Verification items for the finished model (mm, model axes). Round coordinates to 2 decimals unless told otherwise and drop trailing zeros. Order: outer loops, then holes, each group sorted by start corner. A loop starts at its lowest first (then second) coordinate and runs counter-clockwise, first axis right, second up. Notation, with made-up numbers: (45, 81) -> (84, 81) arc R33 cw to (84, 114) -> close; hole circle Ø10 at (-14.75, 15.5). An arc over 180 degrees is marked (long way). Return JSON: item names as keys, results as strings. Group by question number.
1) Scan lines: L1, parallel to Z at x = -3, y = 86.5; L2, parallel to X at y = 77, z = -0.7; L3, parallel to Z at x = 1.5, y = 138.5. Record each from-to range of solid material in increasing order.
2) Depth check by flat-ended pin: pin 1 (2.5 mm diameter, centred on x = 0, y = 155, fed in from -Z); pin 2 (1 mm diameter, centred on y = 116.5, z = -2, fed in from -X); pin 3 (0.5 mm diameter, centred on y = 141, z = -1, fed in from -X). Enter the tip coordinate at first touch or a pass-through.
3) Section check A-A on y = 115.5. Enter the section's corners in (x, z), plus the area to 3 significant figures.
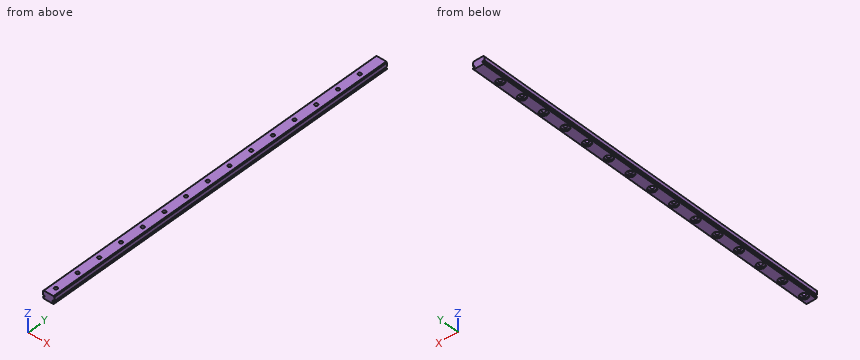
```python
from build123d import *

# Parameters (mm, degrees)
EXTRUDE_1_DEPTH     = 230
SKETCH_2_R          = 1
CUT_EXTRUDE_1_DEPTH = 10
CHAMFER_1_SIZE      = 0.5
SKETCH_3_R          = 2.383304988
CUT_EXTRUDE_2_DEPTH = 1


with BuildPart() as part:
    # 草图1 → 凸台-拉伸1 (new body)
    with BuildSketch(Plane(origin=(0, 0, 0), x_dir=(1, 0, 0), z_dir=(0, 1, 0))):
        Polygon((-3.5, 0.4), (-3.5, -2.4), (3.5, -2.4), (3.5, 0.4), (2.5, 0.4), (2.5, 1.4), (3.5, 1.4), (3.5, 2.4), (-3.5, 2.4), (-3.5, 1.4), (-2.5, 1.4), (-2.5, 0.4), align=None)
    extrude(amount=EXTRUDE_1_DEPTH)

    # 草图2 → 切除-拉伸1 (cut)
    with BuildSketch(Plane(origin=(0, 0, -2.4), x_dir=(-1, 0, 0), z_dir=(0, 0, -1))):
        with Locations((0, 5)):
            Circle(SKETCH_2_R)
        with Locations((0, 20)):
            Circle(SKETCH_2_R)
        with Locations((0, 35)):
            Circle(SKETCH_2_R)
        with Locations((0, 50)):
            Circle(SKETCH_2_R)
        with Locations((0, 65)):
            Circle(SKETCH_2_R)
        with Locations((0, 80)):
            Circle(SKETCH_2_R)
        with Locations((0, 95)):
            Circle(SKETCH_2_R)
        with Locations((0, 110)):
            Circle(SKETCH_2_R)
        with Locations((0, 125)):
            Circle(SKETCH_2_R)
        with Locations((0, 140)):
            Circle(SKETCH_2_R)
        with Locations((0, 155)):
            Circle(SKETCH_2_R)
        with Locations((0, 170)):
            Circle(SKETCH_2_R)
        with Locations((0, 185)):
            Circle(SKETCH_2_R)
        with Locations((0, 200)):
            Circle(SKETCH_2_R)
        with Locations((0, 215)):
            Circle(SKETCH_2_R)
    extrude(amount=-CUT_EXTRUDE_1_DEPTH, mode=Mode.SUBTRACT)

    # 倒角1
    chamfer_1_edges = [part.edges().sort_by_distance(p)[0] for p in [
        (-3.5, 115, -2.4),
        (3.5, 115, -2.4),
        (3.5, 115, 2.4),
        (-3.5, 115, 2.4),
    ]]
    chamfer(chamfer_1_edges, length=CHAMFER_1_SIZE)

    # 草图3 → 切除-拉伸2 (cut)
    with BuildSketch(Plane(origin=(0, 0, -2.4), x_dir=(-1, 0, 0), z_dir=(0, 0, -1))):
        with Locations((0, 5)):
            Circle(SKETCH_3_R)
        with Locations((0, 20)):
            Circle(SKETCH_3_R)
        with Locations((0, 35)):
            Circle(SKETCH_3_R)
        with Locations((0, 50)):
            Circle(SKETCH_3_R)
        with Locations((0, 65)):
            Circle(SKETCH_3_R)
        with Locations((0, 80)):
            Circle(SKETCH_3_R)
        with Locations((0, 95)):
            Circle(SKETCH_3_R)
        with Locations((0, 110)):
            Circle(SKETCH_3_R)
        with Locations((0, 125)):
            Circle(SKETCH_3_R)
        with Locations((0, 140)):
            Circle(SKETCH_3_R)
        with Locations((0, 155)):
            Circle(SKETCH_3_R)
        with Locations((0, 170)):
            Circle(SKETCH_3_R)
        with Locations((0, 185)):
            Circle(SKETCH_3_R)
        with Locations((0, 200)):
            Circle(SKETCH_3_R)
        with Locations((0, 215)):
            Circle(SKETCH_3_R)
    extrude(amount=-CUT_EXTRUDE_2_DEPTH, mode=Mode.SUBTRACT)


solid = part.part
```
Check result:
{
 "1": {"L1": "-2.4 to -1.4, -0.4 to 2.4", "L2": "-2.5 to 2.5", "L3": "-1.4 to 2.4"},
 "2": {"pin 1": "z = -1.4", "pin 2": "x = -3.5", "pin 3": "x = -2.5"},
 "3": {"outline": "(-3.5, -1.9) -> (-3, -2.4) -> (3, -2.4) -> (3.5, -1.9) -> (3.5, -1.4) -> (2.5, -1.4) -> (2.5, -0.4) -> (3.5, -0.4) -> (3.5, 1.9) -> (3, 2.4) -> (-3, 2.4) -> (-3.5, 1.9) -> (-3.5, -0.4) -> (-2.5, -0.4) -> (-2.5, -1.4) -> (-3.5, -1.4) -> close", "area": "31.1 mm^2"}
}
